```python
from build123d import *

# Parameters (mm, degrees)
SKETCH_1_W          = 20
SKETCH_1_H          = 40
SKETCH_1_W_2        = 18
SKETCH_1_H_2        = 38
EXTRUDE_1_DEPTH     = 170
SKETCH_12_R         = 1.6
CUT_EXTRUDE_2_DEPTH = 176.783958312
SKETCH_13_R         = 1.6
CUT_EXTRUDE_3_DEPTH = 176.783958312
SKETCH_14_R         = 1.6
CUT_EXTRUDE_4_DEPTH = 176.783958312


with BuildPart() as part:
    # 草图1 → 凸台-拉伸1 (new body)
    with BuildSketch(Plane.XY):
        with Locations((10, 20)):
            Rectangle(SKETCH_1_W, SKETCH_1_H)
        with Locations((10, 20)):
            Rectangle(SKETCH_1_W_2, SKETCH_1_H_2, mode=Mode.SUBTRACT)
    extrude(amount=EXTRUDE_1_DEPTH)

    # 草图12 → 切除-拉伸2 (cut, through all)
    with BuildSketch(Plane.ZY):
        with Locations((112.92, 7)):
            Circle(SKETCH_12_R)
        with Locations((94.92, 7)):
            Circle(SKETCH_12_R)
        with Locations((76.92, 7)):
            Circle(SKETCH_12_R)
        with Locations((94.92, 23)):
            Circle(SKETCH_12_R)
        with Locations((76.92, 23)):
            Circle(SKETCH_12_R)
        with Locations((112.92, 23)):
            Circle(SKETCH_12_R)
    extrude(amount=-CUT_EXTRUDE_2_DEPTH, mode=Mode.SUBTRACT)

    # 草图13 → 切除-拉伸3 (cut, through all)
    with BuildSketch(Plane.ZY):
        with Locations((163, 29.343081894)):
            Circle(SKETCH_13_R)
        with Locations((163, 10)):
            Circle(SKETCH_13_R)
        with Locations((148.01439139, 29.999994822)):
            Circle(SKETCH_13_R)
        with Locations((148, 10)):
            Circle(SKETCH_13_R)
    extrude(amount=-CUT_EXTRUDE_3_DEPTH, mode=Mode.SUBTRACT)

    # 草图14 → 切除-拉伸4 (cut, through all)
    with BuildSketch(Plane(origin=(0, 40, 0), x_dir=(1, 0, 0), z_dir=(0, 1, 0))):
        with Locations(Location((16, -11, 0), (0, 0, 270))):
            Circle(SKETCH_14_R)
        with Locations(Location((4, -11, 0), (0, 0, 270))):
            Circle(SKETCH_14_R)
        with Locations(Location((16, -5, 0), (0, 0, 270))):
            Circle(SKETCH_14_R)
        with Locations(Location((4, -5, 0), (0, 0, 270))):
            Circle(SKETCH_14_R)
        with Locations(Location((16, -17, 0), (0, 0, 270))):
            Circle(SKETCH_14_R)
        with Locations(Location((4, -17, 0), (0, 0, 270))):
            Circle(SKETCH_14_R)
    extrude(amount=-CUT_EXTRUDE_4_DEPTH, mode=Mode.SUBTRACT)


solid = part.part
```
Design review of the part built by this model. Coordinates are the model's own, in mm. A direction names the side the tool comes from. Coordinates: 2 decimals unless noted, no trailing zeros. Loops run counter-clockwise (first coordinate to the right, second up) from the corner with the lowest first, then second, coordinate; pieces in that order, holes last.
Q1. Tool access review of faces 4 (the face through (1, 20, 84)), 5 (the face through (0.49, 7.07, 111.32)): name each direction out of +Z, -Z, +X, -X, +Y, -Y from which nothing blocks a thin tool from reaching the whole face with its end or side.
Reported:
face 4: +Z, -Z
face 5: +X, -X
Q2. We need section A-A on y = 16. State the section outline as (x, z) points.
Reported:
outline: (0, 0) - (1, 0) - (1, 170) - (0, 170) - close; (19, 0) - (20, 0) - (20, 170) - (19, 170) - close
Q3. The part is to be moulded in two halves that separate along Y. For faces 1 (the face through (0.49, 22.39, 96.4)), 2 (the face through (10, 0, 84)), 3 (the face through (17.08, 39.51, 15.82)), say which applies: +Y half, -Y half, draft (parallel to the pull), parting line (faces both ways), or undercut.
Reported:
face 1: undercut
face 2: -Y half
face 3: draft
Q4. For pin 1 (2.5 mm diameter, centred on y = 30, z = 148.01, fed in from +X); pin 2 (3.5 mm diameter, centred on x = 16, z = 11, fed in from -Y), all flat-tipped, find the tip position at first contact; note any pin that passes through.
Reported:
pin 1: passes through
pin 2: stops at y = 0
Q5. We need section D-D on x = 16. State how many separate pieces and enclosed holes the cut face has, and give its area (3 significant figures).
Reported:
separate pieces: 8
enclosed holes: 0
area: 321 mm2
Q6. We need section B-B on z = 17. State the section outline as (x, y) points.
Reported:
outline: (0, 0) - (2.4, 0) - (2.4, 1) - (1, 1) - (1, 39) - (2.4, 39) - (2.4, 40) - (0, 40) - close; (5.6, 0) - (14.4, 0) - (14.4, 1) - (5.6, 1) - close; (5.6, 39) - (14.4, 39) - (14.4, 40) - (5.6, 40) - close; (17.6, 0) - (20, 0) - (20, 40) - (17.6, 40) - (17.6, 39) - (19, 39) - (19, 1) - (17.6, 1) - close
Q7. We need section C-C on z = 107.5. State the section outline as (x, y) points, and give its area (3 significant figures).
Reported:
outline: (0, 0) - (20, 0) - (20, 40) - (0, 40) - close; hole (1, 1) - (19, 1) - (19, 39) - (1, 39) - close
area: 116 mm2
Q8. To check wall thickness, follow line 1 (X direction, y = 0.3, z = 5); line 2 (Y direction, x = 0.7, z = 112.92); line 3 (Y direction, x = 6.25, z = 51). State the ranges of each line that lie inside material, in increasing order.
Reported:
line 1: x = 0 to 2.4, 5.6 to 14.4, 17.6 to 20
line 2: y = 0 to 5.4, 8.6 to 21.4, 24.6 to 40
line 3: y = 0 to 1, 39 to 40
